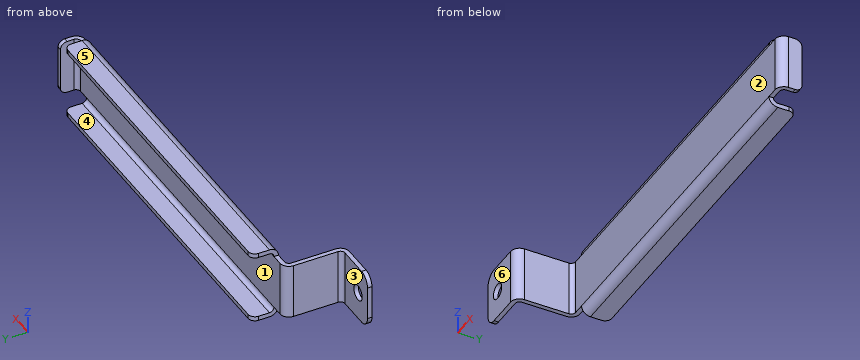
```python
from build123d import *

# Parameters (mm, degrees)
SKETCH_1_W                  = 158
SKETCH_1_H                  = 25
SM_BASE_FLANGE_1_DEPTH      = 2
SM_EDGE_FLANGE_1_DEPTH      = 158
SM_EDGE_FLANGE_1_BEND_DEPTH = 158
SM_EDGE_FLANGE_2_DEPTH      = 25
SM_EDGE_FLANGE_3_DEPTH      = 25
SM_EDGE_FLANGE_4_DEPTH      = 25
FILLET_1_R                  = 3
SKETCH_21_R                 = 3.5
CUT_EXTRUDE_1_DEPTH         = 10
FILLET_2_R                  = 5


# Sheet-metal steps are written as plain solids
with BuildPart() as part:
    # Sketch 1 → Базовая кромка1 (new body)
    with BuildSketch(Plane(origin=(0, 0, 0), x_dir=(1, 0, 0), z_dir=(0, 1, 0))):
        Rectangle(SKETCH_1_W, SKETCH_1_H)
    extrude(amount=-SM_BASE_FLANGE_1_DEPTH)

    # Ребро-кромка1 section (across the edge) → Ребро-кромка1 (add)
    with BuildSketch(Plane(origin=(79, 0, -14.5), x_dir=(0, 0, 1), z_dir=(-1, 0, 0))):
        with BuildLine():
            Line((-2, 2), (-2, 10))
            Line((-2, 10), (0, 10))
            Line((0, 10), (0, 2))
            ThreePointArc((0, 2), (0.585786438, 0.585786438), (2, 0))
            Line((2, 0), (2, -2))
            ThreePointArc((2, -2), (-0.828427125, -0.828427125), (-2, 2))
        make_face()
    extrude(amount=SM_EDGE_FLANGE_1_DEPTH)

    # Ребро-кромка1 section 2 (across the edge) → Ребро-кромка1 bend (add)
    with BuildSketch(Plane(origin=(-79, 0, 14.5), x_dir=(0, 0, -1), z_dir=(1, 0, 0))):
        with BuildLine():
            Line((-2, 2), (-2, 10))
            Line((-2, 10), (0, 10))
            Line((0, 10), (0, 2))
            ThreePointArc((0, 2), (0.585786438, 0.585786438), (2, 0))
            Line((2, 0), (2, -2))
            ThreePointArc((2, -2), (-0.828427125, -0.828427125), (-2, 2))
        make_face()
    extrude(amount=SM_EDGE_FLANGE_1_BEND_DEPTH)

    # Ребро-кромка2 section (across the edge) → Ребро-кромка2 (add)
    with BuildSketch(Plane(origin=(86, 0, 12.5), x_dir=(-1, 0, 0), z_dir=(0, 0, -1))):
        with BuildLine():
            Line((-2, 2), (-2, 8))
            Line((-2, 8), (0, 8))
            Line((0, 8), (0, 2))
            ThreePointArc((0, 2), (0.585786438, 0.585786438), (2, 0))
            Line((2, 0), (7, 0))
            Line((7, 0), (7, -2))
            Line((7, -2), (2, -2))
            ThreePointArc((2, -2), (-0.828427125, -0.828427125), (-2, 2))
        make_face()
    extrude(amount=SM_EDGE_FLANGE_2_DEPTH)

    # Ребро-кромка3 section (across the edge) → Ребро-кромка3 (add)
    with BuildSketch(Plane(origin=(-86, -2, 12.5), x_dir=(1, 0, 0), z_dir=(0, 0, -1))):
        with BuildLine():
            Line((-2, 2), (-2, 22))
            Line((-2, 22), (0, 22))
            Line((0, 22), (0, 2))
            ThreePointArc((0, 2), (0.585786438, 0.585786438), (2, 0))
            Line((2, 0), (7, 0))
            Line((7, 0), (7, -2))
            Line((7, -2), (2, -2))
            ThreePointArc((2, -2), (-0.828427125, -0.828427125), (-2, 2))
        make_face()
    extrude(amount=SM_EDGE_FLANGE_3_DEPTH)

    # Ребро-кромка4 section (across the edge) → Ребро-кромка4 (add)
    with BuildSketch(Plane(origin=(-88, -26, -12.5), x_dir=(0, 1, 0), z_dir=(0, 0, 1))):
        with BuildLine():
            Line((-2, 2), (-2, 21))
            Line((-2, 21), (0, 21))
            Line((0, 21), (0, 2))
            ThreePointArc((0, 2), (0.585786438, 0.585786438), (2, 0))
            Line((2, 0), (2, -2))
            ThreePointArc((2, -2), (-0.828427125, -0.828427125), (-2, 2))
        make_face()
    extrude(amount=SM_EDGE_FLANGE_4_DEPTH)

    # Скругление1
    fillet_1_edges = [part.edges().sort_by_distance(p)[0] for p in [
        (79, 10, -15.5),
        (-79, 10, -15.5),
        (-79, 10, 15.5),
        (79, 10, 15.5),
        (87, 8, 12.5),
        (87, 8, -12.5),
    ]]
    fillet(fillet_1_edges, radius=FILLET_1_R)

    # Эскиз21 → Вырез-Вытянуть1 (cut)
    with BuildSketch(Plane(origin=(0, -26, 0), x_dir=(1, 0, 0), z_dir=(0, 1, 0))):
        with Locations(Location((-101, 0, 0), (0, 0, 270))):
            Circle(SKETCH_21_R)
    extrude(amount=-CUT_EXTRUDE_1_DEPTH, mode=Mode.SUBTRACT)

    # Скругление2
    fillet_2_edges = [part.edges().sort_by_distance(p)[0] for p in [
        (-109, -27, -12.5),
        (-109, -27, 12.5),
    ]]
    fillet(fillet_2_edges, radius=FILLET_2_R)


solid = part.part
```
Geometry: final body of the model. Coordinates: model frame, mm. Face numbers are marked on the shaded views. A direction names the side the tool comes from. Round coordinates to 2 decimals unless told otherwise and drop trailing zeros. Write each loop counter-clockwise with the first axis right and the second up, starting at its lowest first coordinate (ties: lowest second). Pieces come first, ordered by that corner, then holes. Notation, with made-up numbers: (16.25, 86) -> (63.25, 86) arc R19 cw to (63.25, 113) -> close; hole circle Ø2 at (45, 42). An arc over 180 degrees is marked (long way). Return JSON: item names as keys, results as strings.
Q1. Section A-A on z = 0. Return the cut outline in (x, y).
From the geometry:
{"outline": "(-109, -28) -> (-104.5, -28) -> (-104.5, -26) -> (-109, -26) -> close; (-97.5, -28) -> (-90, -28) arc R4 ccw to (-86, -24) -> (-86, -4) arc R2 cw to (-84, -2) -> (84, -2) arc R4 ccw to (88, 2) -> (88, 8) -> (86, 8) -> (86, 2) arc R2 cw to (84, 0) -> (-84, 0) arc R4 ccw to (-88, -4) -> (-88, -24) arc R2 cw to (-90, -26) -> (-97.5, -26) -> close"}
Q2. First-contact query: pin 1 Ø7.5 at (x, y) = (85, 1.5) entering from +Z; pin 2 Ø3.5 at (x, y) = (82.5, 0) entering from -Z; pin 3 Ø4.5 at (y, z) = (4, 14.5) entering from -X. Flat tips, straight axial feed; report the tip coordinate or a pass-through.
From the geometry:
{"pin 1": "z = 12.5", "pin 2": "z = -12.5", "pin 3": "x = -79"}
Q3. Section C-C on x = -15.5. Return the cut outline in (y, z).
From the geometry:
{"outline": "(-2, -12.5) arc R4 ccw to (2, -16.5) -> (10, -16.5) -> (10, -14.5) -> (2, -14.5) arc R2 cw to (0, -12.5) -> (0, 12.5) arc R2 cw to (2, 14.5) -> (10, 14.5) -> (10, 16.5) -> (2, 16.5) arc R4 ccw to (-2, 12.5) -> close"}
Q4. Section B-B on x = -101. Return the cut outline in (y, z), and give its area (3 significant figures).
From the geometry:
{"outline": "(-28, -12.5) -> (-26, -12.5) -> (-26, -3.5) -> (-28, -3.5) -> close; (-28, 3.5) -> (-26, 3.5) -> (-26, 12.5) -> (-28, 12.5) -> close", "area": "36.0 mm2"}
Q5. Mould query, pull axis Z, two halves, no side actions, for the marked faces 4, 5 and 6. Classes: +Z half, -Z half, draft (parallel to the pull), parting line (faces both ways), or undercut.
From the geometry:
{"face 4": "undercut", "face 5": "+Z half", "face 6": "draft"}
Q6. Set-up query: the marked faces 1, 2 and 3. Return all of +Z, -Z, +X, -X, +Y, -Y with unobstructed straight access to the full face (end or side cutting, diameter ignored); none if empty.
From the geometry:
{"face 1": "-X, +Y", "face 2": "+Z, -Z, +X, -Y", "face 3": "+Z, -Z, -X, +Y"}
Q7. Ray query, line 1 (X direction, y = -27.45, z = 0); line 2 (Y direction, x = -5, z = -12); line 3 (X direction, y = -6.5, z = 4). Return the intervals inside material, ascending.
From the geometry:
{"line 1": "-109 to -104.5, -97.5 to -87.98", "line 2": "-2 to 0", "line 3": "-88 to -86"}
